from build123d import *

# Parameters (mm, degrees)
SKETCH1_W           = 60
SKETCH1_H           = 80
BOSS_EXTRUDE1_DEPTH = 50
SKETCH2_W           = 40
SKETCH2_H           = 10
CUT_EXTRUDE1_DEPTH  = 50
CUT_EXTRUDE2_DEPTH  = 30
CUT_EXTRUDE3_DEPTH  = 30
CHAMFER1_SIZE       = 30


with BuildPart() as part:
    # Sketch1 → Boss-Extrude1 (new body)
    with BuildSketch(Plane(origin=(0, 0, 0), x_dir=(1, 0, 0), z_dir=(0, 1, 0))):
        Rectangle(SKETCH1_W, SKETCH1_H)
    extrude(amount=BOSS_EXTRUDE1_DEPTH)

    # Sketch2 → Cut-Extrude1 (cut)
    with BuildSketch(Plane(origin=(0, 50, 0), x_dir=(1, 0, 0), z_dir=(0, 1, 0))):
        with Locations((2.037233821, 35)):
            Rectangle(SKETCH2_W, SKETCH2_H)
    extrude(amount=-CUT_EXTRUDE1_DEPTH, mode=Mode.SUBTRACT)

    # Sketch3 → Cut-Extrude2 (cut)
    with BuildSketch(Plane(origin=(0, 50, 0), x_dir=(1, 0, 0), z_dir=(0, 1, 0))):
        Polygon((0, -10), (30, 10), (30, -40), (0, -40), align=None)
    extrude(amount=-CUT_EXTRUDE2_DEPTH, mode=Mode.SUBTRACT)

    # Sketch4 → Cut-Extrude3 (cut)
    with BuildSketch(Plane(origin=(0, 20, 0), x_dir=(1, 0, 0), z_dir=(0, 1, 0))):
        Polygon((0, -40), (30, -20), (30, -40), align=None)
    extrude(amount=-CUT_EXTRUDE3_DEPTH, mode=Mode.SUBTRACT)

    # Chamfer1
    chamfer1_edges = [part.edges().sort_by_distance(p)[0] for p in [
        (-15, 50, 40),
    ]]
    chamfer(chamfer1_edges, length=CHAMFER1_SIZE)


solid = part.part
Here's how the part is built. I have some questions about the finished solid (model axes, mm). A direction names the side the tool comes from. Round coordinates to 2 decimals unless told otherwise and drop trailing zeros. Loops run counter-clockwise (first coordinate to the right, second up) from the corner with the lowest first, then second, coordinate; pieces in that order, holes last. Notation, with made-up numbers: (6, -3.75) - (13, -3.75) arc R18 ccw to (13, 21.25) - close; hole circle Ø11 at (20.25, 18.25). An arc over 180 degrees is marked (long way). One line per question, with ' | ' between items. Start each with the question number.
Q1. Will these pins go through, and if not, where does the flat tip stop? pin 1 (6 mm diameter, centred on x = 6, y = 13, fed in from -Z); pin 2 (9 mm diameter, centred on y = 32, z = 25, fed in from +X); pin 3 (5 mm diameter, centred on x = -0.5, y = 38.5, fed in from +Z).
Q2. I want a section at D-D (x = -6). Write out the boundary of the cut face in (y, z).
Q3. I want a section at A-A (z = -32). Write out the boundary of the cut face in (x, y).
Q4. We'd pull the mould along X, two halves only. Please class faces 4 (the flat face through (-30, 25, 1)), 5 (the flat face through (-17.963, 25, -35)), 6 (the flat face through (15, 20, 15)), 7 (the flat face through (2, 25, -30)): +X half, -X half, draft (parallel to the pull), parting line (faces both ways), or undercut.
Q5. Please list where these lines run through material, in increasing order: line 1 (Y direction, x = 1, z = 34.5); line 2 (Z direction, x = 0, y = 6); line 3 (X direction, y = 27, z = 17.5). Write a range as [from, to].
Q6. I want a section at C-C (z = 5). Write out the boundary of the cut face in (x, y).
Q7. I want a section at B-B (y = 26.5). Write out the boundary of the cut face in (x, z).
Q8. For faces 1 (the flat face through (15, 35, 0)), 2 (the flat face through (22.037, 25, -35)), 3 (the flat face through (26, 25, -40)), which set-ups out of +Z, -Z, +X, -X, +Y, -Y let a thin tool reach every point of the face, with its end or its side?
Response values:
1) pin 1: stops at z = -30 | pin 2: stops at x = 0 | pin 3: stops at z = 24
2) outline: (0, -30) - (50, -30) - (50, 10) - (20, 40) - (0, 40) - close
3) outline: (-30, 0) - (-17.96, 0) - (-17.96, 50) - (-30, 50) - close; (22.04, 0) - (30, 0) - (30, 50) - (22.04, 50) - close
4) face 4: -X half | face 5: undercut | face 6: draft | face 7: undercut
5) line 1: y = [0, 20] | line 2: z = [-30, 40] | line 3: x = [-30, 0]
6) outline: (-30, 0) - (30, 0) - (30, 20) - (7.5, 20) - (7.5, 50) - (-30, 50) - close
7) outline: (-30, -40) - (-17.96, -40) - (-17.96, -30) - (22.04, -30) - (22.04, -40) - (30, -40) - (30, -10) - (0, 10) - (0, 33.5) - (-30, 33.5) - close
8) face 1: +Z, +X, +Y | face 2: -Z, +Y, -Y | face 3: -Z, +X, -X, +Y, -Y
